Geometry check sheet. Reference: the model listing, model coordinates, mm. Round coordinates to 2 decimals unless told otherwise and drop trailing zeros. Order: outer loops, then holes, each group sorted by start corner. A loop starts at its lowest first (then second) coordinate and runs counter-clockwise, first axis right, second up. Notation, with made-up numbers: (11.25, -8) -> (53.25, -8) arc R28 ccw to (53.25, 28) -> close; hole circle Ø11 at (64, 35). An arc over 180 degrees is marked (long way). Use a Markdown table: item, result. Add a question column.
Item 1: Sectioned sample at C-C, the plane z = -111. Record the cut outline in (x, y).
Item 2: Material ranges on probe 1 along Z at (x, y) = (44, 5); probe 2 along X at (y, z) = (4.25, -112.5); probe 3 along Z at (x, y) = (86.5, 0.5), recorded low to high. Write a range as [from, to].
Item 3: Sectioned sample at A-A, the plane y = 1.5. State how many separate pieces and enclosed holes the cut face has, and give its area (4 significant figures).
Item 4: Sectioned sample at B-B, the plane x = -17. Record the cut outline in (y, z).
Item 5: Gauge pin test, flat ends, axial feed: pin 1 Ø1 at (y, z) = (1.5, -14) entering from +X; pin 2 Ø5 at (x, z) = (38.9, -0.21) entering from +Y; pin 3 Ø1 at (y, z) = (5.5, -22) entering from -X; pin 4 Ø2 at (y, z) = (5, -111) entering from -X. Record the tip position at first contact, or that the pin passes through.
Item 6: Mould release check, pull along Z, two halves, no side actions. Record for faces 1 (the cylindrical face through (201.94, 3.13, -156.21)), 2 (the flat face through (142.73, 3.13, -73.57)), 3 (the flat face through (-3, 3, -9.739)): pulls with the +Z half, pulls with the -Z half, needs draft (parallel to the pull), parting line crosses it, or undercut.
from build123d import *

# Parameters (mm, degrees)
SKETCH2_R           = 2.6035
SKETCH2_R_2         = 2.667
BOSS_EXTRUDE1_DEPTH = 6.35


with BuildPart() as part:
    # Sketch2 → Boss-Extrude1 (new body)
    with BuildSketch(Plane(origin=(0, 0, 0), x_dir=(1, 0, 0), z_dir=(0, 1, 0))):
        with BuildLine():
            Line((68.109325708, 14.275642301), (192.061641465, 161.996259914))
            ThreePointArc((192.061641465, 161.996259914), (205.480766768, 163.170281253), (206.654788106, 149.75115595))
            Line((206.654788106, 149.75115595), (76.992486596, -4.774357699))
            ThreePointArc((76.992486596, -4.774357699), (72.630974093, -8.121063952), (67.263722169, -9.310955056))
            Line((67.263722169, -9.310955056), (64.302668539, -9.310955056))
            Line((64.302668539, -9.310955056), (-62.697331461, -9.310955056))
            ThreePointArc((-62.697331461, -9.310955056), (-72.222331461, 0.214044944), (-62.697331461, 9.739044944))
            Line((-62.697331461, 9.739044944), (58.380561281, 9.739044944))
            ThreePointArc((58.380561281, 9.739044944), (63.747813205, 10.928936048), (68.109325708, 14.275642301))
        make_face()
        with Locations(Location((-62.697331461, 0.214044944, 0), (0, 0, 270))):
            Circle(SKETCH2_R, mode=Mode.SUBTRACT)
        with Locations(Location((199.358214786, 155.873707932, 0), (0, 0, 270))):
            Circle(SKETCH2_R, mode=Mode.SUBTRACT)
        with Locations(Location((38.902668539, 0.214044944, 0), (0, 0, 270))):
            Circle(SKETCH2_R_2, mode=Mode.SUBTRACT)
    extrude(amount=BOSS_EXTRUDE1_DEPTH)


solid = part.part
Found:
| question | item | result |
|---|---|---|
| 1 | outline | (149.27, 0) -> (174.14, 0) -> (174.14, 6.35) -> (149.27, 6.35) -> close |
| 2 | probe 1 | z = [-9.74, 9.31] |
| 2 | probe 2 | x = [150.53, 175.4] |
| 2 | probe 3 | z = [-36.19, -6.56] |
| 3 | separate pieces | 1 |
| 3 | enclosed holes | 3 |
| 3 | area | 6,595 mm2 |
| 4 | outline | (0, -9.74) -> (6.35, -9.74) -> (6.35, 9.31) -> (0, 9.31) -> close |
| 5 | pin 1 | stops at x = 93.17 |
| 5 | pin 2 | passes through |
| 5 | pin 3 | stops at x = 74.17 |
| 5 | pin 4 | stops at x = 148.43 |
| 6 | face 1 | undercut |
| 6 | face 2 | pulls with the +Z half |
| 6 | face 3 | pulls with the -Z half |
